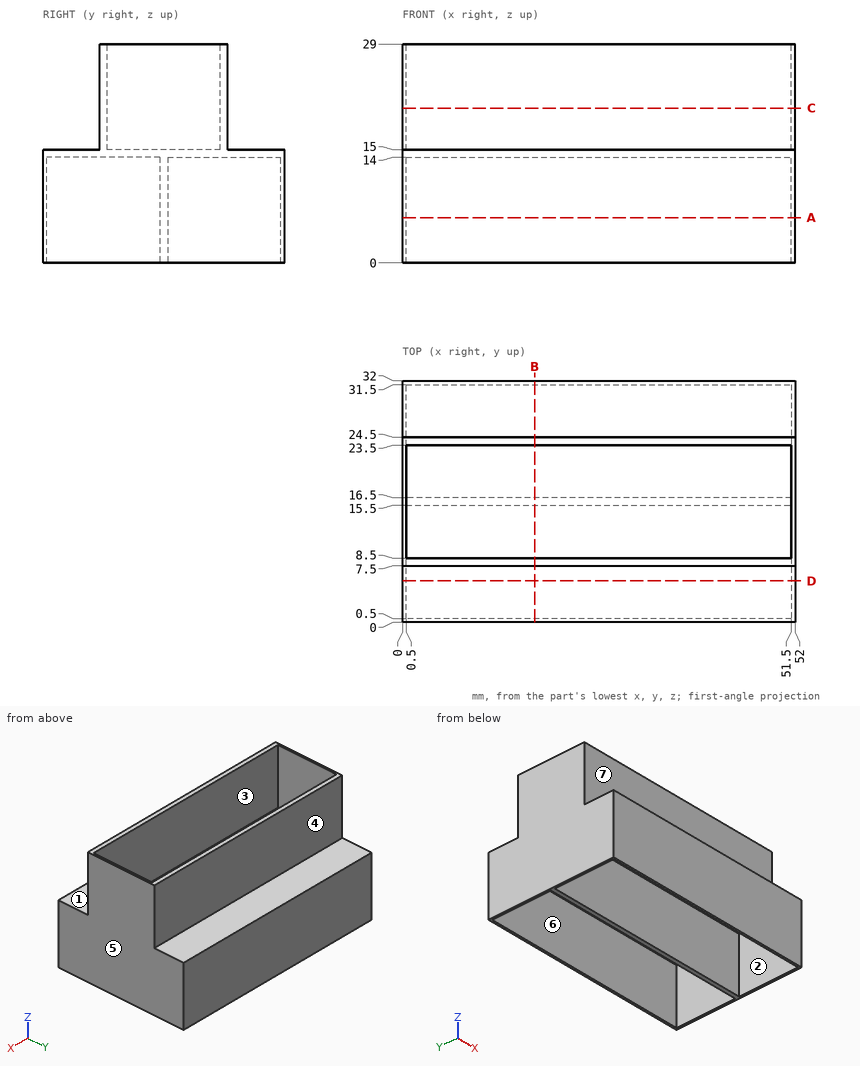
For this review, use the dimensioned drawing (mm, ordinates from the lowest corner) and the shaded views. A direction names the side the tool comes from. Round coordinates to 2 decimals unless told otherwise and drop trailing zeros. Write each loop counter-clockwise with the first axis right and the second up, starting at its lowest first coordinate (ties: lowest second). Pieces come first, ordered by that corner, then holes. Notation, with made-up numbers: M 9.25,74.5 L 43.25,74.5 A27 ccw 43.25,107.5 Z; hole C -22.75,76.25 d8. An arc over 180 degrees is marked long. Answer as CSV lines item,"result". Start each with the question number.
Q1. Clearance check with flat-ended pins moving along their axes: P1, Ø7, axis at x = 17, z = 22.5, coming from the +Y side; P2, Ø7, axis at x = 15, z = 22, coming from the -Y side; P3, Ø4.5, axis at x = 16, y = 21, coming from the -Z side. State where each tip first meets the part, or that it passes through.
Q2. Consider section C-C, the plane z = 20.5. Give the boundary of the cut face in (x, y).
Q3. The part is to be moulded in two halves that separate along X. For the marked faces 5, 6 and 7, say which applies: +X half, -X half, draft (parallel to the pull), parting line (faces both ways), or undercut.
Q4. Consider section A-A, the plane z = 6. Give the boundary of the cut face in (x, y), then the cut area to 3 significant figures.
Q5. Consider section B-B, the plane x = 17.5. Give the boundary of the cut face in (y, z), then the cut area to 3 significant figures.
Q6. Tool access review of the marked faces 1, 2, 3 and 4: name each direction out of +Z, -Z, +X, -X, +Y, -Y from which nothing blocks a thin tool from reaching the whole face with its end or side.
Q7. Wall thickness on line 1 along Y through (x, z) = (8.5, 8); line 2 along X through (y, z) = (20, 7); line 3 along Y through (x, z) = (38, 19.5): over which ranges is each line inside the solid? List them lowest first.
Q8. Consider section D-D, the plane y = 5.5. Give the boundary of the cut face in (x, z).
Result set:
1,P1,"stops at y = 24.5"
1,P2,"stops at y = 7.5"
1,P3,"stops at z = 14"
2,outline,"M 0,7.5 L 52,7.5 L 52,24.5 L 0,24.5 Z; hole M 0.5,8.5 L 51.5,8.5 L 51.5,23.5 L 0.5,23.5 Z"
3,face 5,"+X half"
3,face 6,"undercut"
3,face 7,"draft"
4,outline,"M 0,0 L 52,0 L 52,32 L 0,32 Z; hole M 0.5,0.5 L 51.5,0.5 L 51.5,15.5 L 0.5,15.5 Z; hole M 0.5,16.5 L 51.5,16.5 L 51.5,31.5 L 0.5,31.5 Z"
4,area,"134 mm²"
5,outline,"M 0,0 L 0.5,0 L 0.5,14 L 15.5,14 L 15.5,0 L 16.5,0 L 16.5,14 L 31.5,14 L 31.5,0 L 32,0 L 32,15 L 24.5,15 L 24.5,29 L 23.5,29 L 23.5,15 L 8.5,15 L 8.5,29 L 7.5,29 L 7.5,15 L 0,15 Z"
5,area,"88.0 mm²"
6,face 1,"+Z, +X, -X, -Y"
6,face 2,"-Z"
6,face 3,"+Z"
6,face 4,"+Z, +X, -X, +Y"
7,line 1,"y = 0 to 0.5, 15.5 to 16.5, 31.5 to 32"
7,line 2,"x = 0 to 0.5, 51.5 to 52"
7,line 3,"y = 7.5 to 8.5, 23.5 to 24.5"
8,outline,"M 0,0 L 0.5,0 L 0.5,14 L 51.5,14 L 51.5,0 L 52,0 L 52,15 L 0,15 Z"
